The listing builds one solid part. Answer for the finished solid, in the listing's coordinates (mm). A direction names the side the tool comes from. Give positions to 0.01 mm unless a question says otherwise; leave off trailing zeros. Write each loop counter-clockwise with the first axis right and the second up, starting at its lowest first coordinate (ties: lowest second). Pieces come first, ordered by that corner, then holes. Notation, with made-up numbers: (55, -24.75) - (83, -24.75) arc R27 ccw to (83, 10.25) - close; hole circle Ø7 at (32, 32.25). An arc over 180 degrees is marked (long way). Answer as CSV lines item,"result". Start each with the question number.
(1) Find section D-D (y = -5.25). Write down the section's boundary in (x, z) (3 decimals).
(2) Find section C-C (x = 5.5). Write down the section's boundary in (y, z) (3 decimals).
(3) Each of these flat-tipped pins is pushed along its axis until it touches: pin 1 Ø3 at (x, z) = (-0.5, 32.5) entering from -Y; pin 2 Ø3 at (x, z) = (5, 30) entering from -Y; pin 3 Ø4 at (x, y) = (0, 0) entering from -Z; pin 4 Ø1.1 at (x, y) = (0.5, 7) entering from -Z (3 decimals). Where does it stop, or does it pass through?
(4) For a pull along X with two mould halves and no side action, classify faces 5 (the face through (3, 0, 0)), 6 (the face through (0, 2.195, 39)), 7 (the face through (1.588, 7, 40)) as pulls with the +X half, pulls with the -X half, needs draft (parallel to the pull), parting line crosses it, or undercut.
(5) Straight lines are drawn through the part: probe 1 along Y at (x, z) = (0, 41.5) (3 decimals); probe 2 along X at (y, z) = (0, 16.5) (3 decimals); probe 3 along Y at (x, z) = (0, 60.5) (3 decimals). For each, find the intervals that lie inside material, in ascending order.
(6) For faces 1 (the face through (0.093, -2.573, 39.44)), 2 (the face through (-5.08, -3.89, 75.97)), 3 (the face through (-1.588, 7, 40)), 4 (the face through (-3, -6, 54.275)), determine the directions among +Z, -Z, +X, -X, +Y, -Y from which every point of the face is accessible in a straight line to the end or side of a thin tool.
(7) Find section A-A (y = 0). Write down the section's boundary in (x, z) (3 decimals), then the cut area to 3 significant figures.
from build123d import *

# Parameters (mm, degrees)
SKETCH1_R                = 6.4
BOSS_EXTRUDE1_DEPTH      = 80
BOSS_EXTRUDE2_DEPTH      = 14.275
BOSS_EXTRUDE2_DEPTH_BACK = 14.275
SKETCH9_W                = 3.175
SKETCH9_H                = 4
BOSS_EXTRUDE3_START      = -7.9502
SKETCH10_R               = 7.5819
SKETCH10_R_2             = 5
BOSS_EXTRUDE3_DEPTH      = 17.7748


with BuildPart() as part:
    # Sketch1 → Boss-Extrude1 (new body)
    with BuildSketch(Plane.XY):
        Circle(SKETCH1_R)
        with BuildLine():
            Line((-1.34632834, 2.195), (1.34632834, 2.195))
            ThreePointArc((1.34632834, 2.195), (0, -2.575), (-1.34632834, 2.195))
        make_face(mode=Mode.SUBTRACT)
    extrude(amount=BOSS_EXTRUDE1_DEPTH)

    # Sketch9 → Boss-Extrude2 (add, two sides: drawn at the far end of the back side and taken through both)
    with BuildSketch(Plane.XY.offset(40).offset(-BOSS_EXTRUDE2_DEPTH_BACK)):
        with Locations((0, 5.5819)):
            Rectangle(SKETCH9_W, SKETCH9_H)
    extrude(amount=BOSS_EXTRUDE2_DEPTH + BOSS_EXTRUDE2_DEPTH_BACK)

    # Sketch10 → Boss-Extrude3 (add)
    with BuildSketch(Plane.XY.offset(80).offset(BOSS_EXTRUDE3_START)):
        Circle(SKETCH10_R)
        Circle(SKETCH10_R_2, mode=Mode.SUBTRACT)
    extrude(amount=-BOSS_EXTRUDE3_DEPTH)


solid = part.part
Result set:
1,outline,"(-5.47, 54.275) - (-3.66, 54.275) - (-3.66, 0) - (3.66, 0) - (3.66, 54.275) - (5.47, 54.275) - (5.47, 72.05) - (3.66, 72.05) - (3.66, 80) - (-3.66, 80) - (-3.66, 72.05) - (-5.47, 72.05) - close"
2,outline,"(-5.219, 54.275) - (-3.273, 54.275) - (-3.273, 0) - (3.273, 0) - (3.273, 54.275) - (5.219, 54.275) - (5.219, 72.05) - (3.273, 72.05) - (3.273, 80) - (-3.273, 80) - (-3.273, 72.05) - (-5.219, 72.05) - close"
3,pin 1,"y = -6.4"
3,pin 2,"y = -5.36"
3,pin 3,"through"
3,pin 4,"z = 25.725"
4,face 5,"needs draft"
4,face 6,"undercut"
4,face 7,"pulls with the +X half"
5,probe 1,"-6.4 to -2.575, 2.195 to 7.582"
5,probe 2,"-6.4 to -2.575, 2.575 to 6.4"
5,probe 3,"-7.582 to -2.575, 2.195 to 7.582"
6,face 1,"+Z, -Z"
6,face 2,"+Z"
6,face 3,"-Z, -X, +Y"
6,face 4,"-Z"
7,outline,"(-7.582, 54.275) - (-6.4, 54.275) - (-6.4, 0) - (-2.575, 0) - (-2.575, 80) - (-6.4, 80) - (-6.4, 72.05) - (-7.582, 72.05) - close; (2.575, 0) - (6.4, 0) - (6.4, 54.275) - (7.582, 54.275) - (7.582, 72.05) - (6.4, 72.05) - (6.4, 80) - (2.575, 80) - close"
7,area,"654 mm^2"
